```python
from build123d import *

# Parameters (mm, degrees)
F0_W     = 90
F0_H     = 60
F1_DEPTH = 100
F3_W     = 84
F3_H     = 54
F4_DEPTH = 95
F5_R     = 27.5
F6_DEPTH = 3


with BuildPart() as f1:
    # F0 (on Top) → F1 (new body)
    with BuildSketch(Plane.XY):
        with Locations((45, -30)):
            Rectangle(F0_W, F0_H)
    extrude(amount=F1_DEPTH)

    # F3 (on offset) → F4 (cut, through all)
    with BuildSketch(Plane.XY.offset(95)):
        with Locations((45, -30)):
            Rectangle(F3_W, F3_H)
    extrude(amount=-F4_DEPTH, mode=Mode.SUBTRACT)

    # F5 (on face) → F6 (cut, through all)
    with BuildSketch(Plane.XZ.offset(60)):
        with Locations((45, 40)):
            Circle(F5_R)
    extrude(amount=-F6_DEPTH, mode=Mode.SUBTRACT)


solid = f1.part
```
CAD build for the part. Positions are in the model's coordinates, mm. A direction names the side the tool comes from. Round coordinates to 2 decimals unless told otherwise and drop trailing zeros. Order: outer loops, then holes, each group sorted by start corner. A loop starts at its lowest first (then second) coordinate and runs counter-clockwise, first axis right, second up. Notation, with made-up numbers: (-39, 49.25) - (-8, 49.25) arc R17 cw to (-8, 68.25) - close; hole circle Ø5 at (-28.5, -15). An arc over 180 degrees is marked (long way). Answer as CSV lines item,"result". Start each with the question number.
1. Drill centre lines: L1, parallel to Z at x = 45, y = -59.3; L2, parallel to Y at x = 4, z = 11.5; L3, parallel to X at y = -50, z = 44. Where is each one in solid material? Low to high. Write a range as [from, to].
2. Saw through at C-C, the plane y = -31.5. Write the cut outline in (x, z).
3. Saw through at B-B, the plane x = 45. Write the cut outline in (y, z), and give its area (3 significant figures).
4. Pin check, flat tips, straight feed: pin 1 (3 mm diameter, centred on x = 20, y = -50, fed in from -Z); pin 2 (4 mm diameter, centred on x = 50, z = 44, fed in from -Y). Stop position of each tip, or through.
5. Saw through at A-A, the plane z = 7.5. Write the cut outline in (x, y).
6. Tool access for faces 1 (the face through (44, -30, 95)), 2 (the face through (44, 0, 49)), 3 (the face through (17.527, -58.521, 41.209)): list every direction of +Z, -Z, +X, -X, +Y, -Y with a clear straight run to the whole face (end or side of a thin tool).
7. Saw through at D-D, the plane z = 40. Write the cut outline in (x, y), and give its area (3 significant figures).
8. Pull direction X, two halves, no side cores. Call faces 4 (the face through (0, -30, 49)), 5 (the face through (3, -30, 48)), 6 (the face through (90, -30, 49)): +X half, -X half, draft (parallel to the pull), parting line (faces both ways), or undercut.
Model answer:
1,L1,"z = [0, 12.5], [67.5, 100]"
1,L2,"y = [-60, -57], [-3, 0]"
1,L3,"x = [0, 3], [87, 90]"
2,outline,"(0, 0) - (3, 0) - (3, 95) - (87, 95) - (87, 0) - (90, 0) - (90, 100) - (0, 100) - close"
3,outline,"(-60, 0) - (-57, 0) - (-57, 12.5) - (-60, 12.5) - close; (-60, 67.5) - (-57, 67.5) - (-57, 95) - (-3, 95) - (-3, 0) - (0, 0) - (0, 100) - (-60, 100) - close"
3,area,"705 mm²"
4,pin 1,"stops at z = 95"
4,pin 2,"stops at y = -3"
5,outline,"(0, -60) - (90, -60) - (90, 0) - (0, 0) - close; hole (3, -57) - (87, -57) - (87, -3) - (3, -3) - close"
6,face 1,"-Z"
6,face 2,"+Z, -Z, +X, -X, +Y"
6,face 3,"-Y"
7,outline,"(0, -60) - (17.5, -60) - (17.5, -57) - (3, -57) - (3, -3) - (87, -3) - (87, -57) - (72.5, -57) - (72.5, -60) - (90, -60) - (90, 0) - (0, 0) - close"
7,area,"699 mm²"
8,face 4,"-X half"
8,face 5,"undercut"
8,face 6,"+X half"
